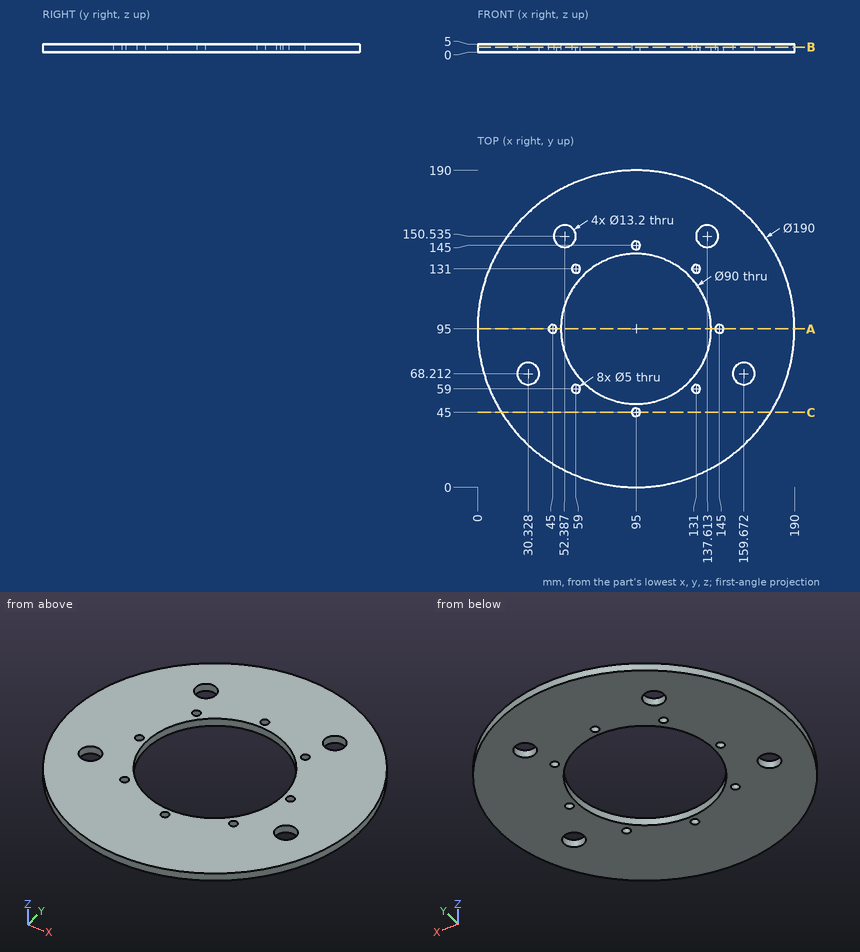
Check sheet for the drawn part. Datum: minimum x, y, z corner. Units: mm. Round coordinates to 2 decimals unless told otherwise and drop trailing zeros. Order: outer loops, then holes, each group sorted by start corner. A loop starts at its lowest first (then second) coordinate and runs counter-clockwise, first axis right, second up.
1. Section check C-C on y = 45. Record the cut outline in (x, z).
Final values:
outline: (14.22, 0) - (92.5, 0) - (92.5, 5) - (14.22, 5) - close; (97.5, 0) - (175.78, 0) - (175.78, 5) - (97.5, 5) - close
2. Section check B-B on z = 3.2. State how many separate pieces and enclosed holes the cut face has, then the cut area to 3 significant figures.
Final values:
separate pieces: 1
enclosed holes: 13
area: 21,300 mm2
3. Section check A-A on y = 95. Record the cut outline in (x, z), then the cut area to 3 significant figures.
Final values:
outline: (0, 0) - (42.5, 0) - (42.5, 5) - (0, 5) - close; (47.5, 0) - (50, 0) - (50, 5) - (47.5, 5) - close; (140, 0) - (142.5, 0) - (142.5, 5) - (140, 5) - close; (147.5, 0) - (190, 0) - (190, 5) - (147.5, 5) - close
area: 450 mm2
4. Go/stop test with flat-tipped pins: P1, Ø4.5, axis at x = 131, y = 131, coming from the -Z side; P2, Ø1, axis at x = 110, z = 3.5, coming from the +Y side; P3, Ø1.5, axis at x = 29.5, z = 2.5, coming from the +Y side (1 decimal). Record where each tip stops, or that it passes through.
Final values:
P1: passes through
P2: stops at y = 188.89
P3: stops at y = 164.5
5. Thickness scan on L1, parallel to Y at x = 95, z = 3.95; L2, parallel to X at y = 150.5, z = 4.55 (1 decimal); L3, parallel to X at y = 131, z = 1.8 (1 decimal). Record the ranges inside material, lowest first.
Final values:
L1: y = 0 to 42.5, 47.5 to 50, 140 to 142.5, 147.5 to 190
L2: x = 17.9 to 45.8, 59 to 131, 144.2 to 172.1
L3: x = 7.1 to 56.5, 61.5 to 68, 122 to 128.5, 133.5 to 182.9
